Autodesk Fusion 360 part; units mm, degrees
sketch "Sketch1" plane through (0, 0, 0) normal (0, 1, 0) x (1, 0, 0)
  circle A0 centre (0, 0) radius 14
  dimension "d1" = 28
extrude "Extrude1" add sketch "Sketch1" along normal blind 38.333
fillet "Fillet1" radius 0.5 1 edges at (-13.0526, 0, 5.0626)
sketch "Sketch2" plane through (0, 0, 0) normal (0, -1, 0) x (1, 0, 0)
  circle A0 centre (0, 0) radius 13.5
  circle A1 centre (0, 0) radius 3.5
  dimension "d6" = 7
extrude "Extrude2" add sketch "Sketch2" along normal blind 37.67 contours A1
CAD build for the part. Positions are in the model's coordinates, mm. A direction names the side the tool comes from. Coordinates: 2 decimals unless noted, no trailing zeros. Write each loop counter-clockwise with the first axis right and the second up, starting at its lowest first coordinate (ties: lowest second). Pieces come first, ordered by that corner, then holes. Notation, with made-up numbers: M -4.5,14.5 L 10.5,14.5 A18 cw 10.5,47.5 Z; hole C 67.25,-12 d9. An arc over 180 degrees is marked long. Return JSON: item names as keys, results as strings.
Item 1: Slice it at C-C, the plane y = -29.5. Write the cut outline in (x, z).
Findings below:
{"outline": "C 0,0 d7"}
Item 2: Which spindle directions (+Z, -Z, +X, -X, +Y, -Y) get a long thin tool onto all of the face, cutting with end or side? Do faces 1 (the flat face through (3, 0, 3)), 2 (the cylindrical face through (12.932, 19.152, -5.362)). Say none if no direction does.
Findings below:
{"face 1": "-Y", "face 2": "+Y, -Y"}
Item 3: Drop flat-ended pins along their axis: pin 1 Ø1 at (x, y) = (3, 26.5) entering from +Z (3 decimals); pin 2 Ø4 at (x, y) = (-4, 0) entering from -Z; pin 3 Ø1 at (y, z) = (-28.5, 2.5) entering from -X; pin 4 Ø5 at (y, z) = (-15, -6.5) entering from +X. Give the stop position or say it passes through.
Findings below:
{"pin 1": "stops at z = 13.775", "pin 2": "stops at z = -13.85", "pin 3": "stops at x = -2.87", "pin 4": "passes through"}
Item 4: Slice it at D-D, the plane y = 30. Write the cut outline in (x, z).
Findings below:
{"outline": "C 0,0 d28"}
Item 5: Slice it at B-B, the plane z = 0. Write the cut outline in (x, y).
Findings below:
{"outline": "M -14,0.5 A0.5 ccw -13.5,0 L -3.5,0 L -3.5,-37.67 L 3.5,-37.67 L 3.5,0 L 13.5,0 A0.5 ccw 14,0.5 L 14,38.33 L -14,38.33 Z"}
Item 6: Probe line 1 (Y direction, x = -4, z = 10.5); line 2 (Z direction, x = 3.75, y = 32); line 3 (X direction, y = -25.5, z = -1). List the from-to ranges inside material, lowest first. Write a range as from..to.
Findings below:
{"line 1": "y = 0..38.33", "line 2": "z = -13.49..13.49", "line 3": "x = -3.35..3.35"}
Item 7: Slice it at A-A, the plane x = 0. Write the cut outline in (y, z), and give its area (3 significant figures).
Findings below:
{"outline": "M -37.67,-3.5 L 0,-3.5 L 0,-13.5 A0.5 ccw 0.5,-14 L 38.33,-14 L 38.33,14 L 0.5,14 A0.5 ccw 0,13.5 L 0,3.5 L -37.67,3.5 Z", "area": "1,340 mm2"}
